The model under review builds one solid part; all positions refer to its coordinate system, in mm. A direction names the side the tool comes from. Give positions to 0.01 mm unless a question says otherwise; leave off trailing zeros. Loops run counter-clockwise (first coordinate to the right, second up) from the corner with the lowest first, then second, coordinate; pieces in that order, holes last. Notation, with made-up numbers: M 20,81 L 73,81 A21 cw 73,96 Z; hole C -18.5,72 d7. An arc over 180 degrees is marked long. Put each result on its own line as item: value. Start each with the question number.
from build123d import *

# Parameters (mm, degrees)
F0_W     = 2145
F0_H     = 1470
F0_W_2   = 655
F0_H_2   = 1042.5
F0_H_3   = 292.5
F1_DEPTH = 50
F2_W     = 15
F2_H     = 292.5
F3_DEPTH = 20


with BuildPart() as f1:
    # F0 (on Front) → F1 (new body)
    with BuildSketch(Plane.XZ):
        with Locations((1072.5, 735)):
            Rectangle(F0_W, F0_H)
        with Locations((372.5, 566.25)):
            Rectangle(F0_W_2, F0_H_2, mode=Mode.SUBTRACT)
        with Locations((1072.5, 566.25)):
            Rectangle(F0_W_2, F0_H_2, mode=Mode.SUBTRACT)
        with Locations((1772.5, 566.25)):
            Rectangle(F0_W_2, F0_H_2, mode=Mode.SUBTRACT)
        with Locations((372.5, 1278.75)):
            Rectangle(F0_W_2, F0_H_3, mode=Mode.SUBTRACT)
        with Locations((1072.5, 1278.75)):
            Rectangle(F0_W_2, F0_H_3, mode=Mode.SUBTRACT)
        with Locations((1772.5, 1278.75)):
            Rectangle(F0_W_2, F0_H_3, mode=Mode.SUBTRACT)
    extrude(amount=F1_DEPTH)

    # F2 (on Front) → F3 (join)
    with BuildSketch(Plane.XZ):
        Polygon((365, 750), (45, 750), (45, 735), (365, 735), (365, 397.5), (45, 397.5), (45, 382.5), (365, 382.5), (365, 45), (380, 45), (380, 382.5), (700, 382.5), (700, 397.5), (380, 397.5), (380, 735), (700, 735), (700, 750), (380, 750), (380, 1087.5), (365, 1087.5), align=None)
        with Locations((372.5, 1278.75)):
            Rectangle(F2_W, F2_H)
        with Locations((1072.5, 1278.75)):
            Rectangle(F2_W, F2_H)
        Polygon((1065, 750), (745, 750), (745, 735), (1065, 735), (1065, 397.5), (745, 397.5), (745, 382.5), (1065, 382.5), (1065, 45), (1080, 45), (1080, 382.5), (1400, 382.5), (1400, 397.5), (1080, 397.5), (1080, 735), (1400, 735), (1400, 750), (1080, 750), (1080, 1087.5), (1065, 1087.5), align=None)
        with Locations((1772.5, 1278.75)):
            Rectangle(F2_W, F2_H)
        Polygon((1780, 1087.5), (1765, 1087.5), (1765, 750), (1445, 750), (1445, 735), (1765, 735), (1765, 397.5), (1445, 397.5), (1445, 382.5), (1765, 382.5), (1765, 45), (1780, 45), (1780, 382.5), (2100, 382.5), (2100, 397.5), (1780, 397.5), (1780, 735), (2100, 735), (2100, 750), (1780, 750), align=None)
    extrude(amount=F3_DEPTH)


solid = f1.part
(1) Insertion check: pin 1 (12 mm diameter, centred on x = 1775, z = 1219.5, fed in from -Y). The pin has a flat end and moves straight along its axis. Give the tip position at first contact, or say it passes through.
(2) For faces 1 (the flat face through (745, -25, 1277)), 2 (the flat face through (1067, -50, 1120)), 3 (the flat face through (1771, -20, 569)), list the 3-axis set-ups (+Z, -Z, +X, -X, +Y, -Y) from which the entire face can be reached by the end or side of a thin tool; tool diameter is ignored.
(3) To check wall thickness, follow L1, parallel to X at y = -45.5, z = 495.5; L2, parallel to Z at x = 1930.5, y = -5; L3, parallel to Z at x = 406, y = -26.5. State the ranges of each line that lie inside material, in increasing order. Write a range as [from, to].
(4) We need section C-C, the plane y = -36. Write out the cut boundary in (x, z), plus the area to 3 significant figures.
(5) We need section A-A, the plane x = 519. Write out the cut boundary in (y, z), plus the area to 3 significant figures.
(6) Draft analysis for pull direction X (two halves, no side actions). For faces 4 (the flat face through (1068, -25, 1132.5)), 5 (the flat face through (1067, 0, 684)), 6 (the flat face through (1768, -25, 1087.5)), state which applies: +X half, -X half, draft (parallel to the pull), parting line (faces both ways), or undercut.
(7) We need section B-B, the plane z = 297.5. Write out the cut boundary in (x, y).
Check sheet entries:
1. pin 1: stops at y = -20
2. face 1: +Y, -Y
2. face 2: +Z, -Z, +X, -X, -Y
2. face 3: -Y
3. L1: x = [0, 45], [700, 745], [1400, 1445], [2100, 2145]
3. L2: z = [0, 45], [382.5, 397.5], [735, 750], [1087.5, 1132.5], [1425, 1470]
3. L3: z = [0, 45], [1087.5, 1132.5], [1425, 1470]
4. outline: M 0,0 L 2145,0 L 2145,1470 L 0,1470 Z; hole M 45,45 L 700,45 L 700,1087.5 L 45,1087.5 Z; hole M 45,1132.5 L 700,1132.5 L 700,1425 L 45,1425 Z; hole M 745,45 L 1400,45 L 1400,1087.5 L 745,1087.5 Z; hole M 745,1132.5 L 1400,1132.5 L 1400,1425 L 745,1425 Z; hole M 1445,45 L 2100,45 L 2100,1087.5 L 1445,1087.5 Z; hole M 1445,1132.5 L 2100,1132.5 L 2100,1425 L 1445,1425 Z
4. area: 530,000 mm²
5. outline: M -50,0 L 0,0 L 0,45 L -50,45 Z; M -50,1087.5 L 0,1087.5 L 0,1132.5 L -50,1132.5 Z; M -50,1425 L 0,1425 L 0,1470 L -50,1470 Z; M -20,382.5 L 0,382.5 L 0,397.5 L -20,397.5 Z; M -20,735 L 0,735 L 0,750 L -20,750 Z
5. area: 7,350 mm²
6. face 4: undercut
6. face 5: draft
6. face 6: undercut
7. outline: M 0,-50 L 45,-50 L 45,0 L 0,0 Z; M 365,-20 L 380,-20 L 380,0 L 365,0 Z; M 700,-50 L 745,-50 L 745,0 L 700,0 Z; M 1065,-20 L 1080,-20 L 1080,0 L 1065,0 Z; M 1400,-50 L 1445,-50 L 1445,0 L 1400,0 Z; M 1765,-20 L 1780,-20 L 1780,0 L 1765,0 Z; M 2100,-50 L 2145,-50 L 2145,0 L 2100,0 Z
